```python
from build123d import *

# Parameters (mm, degrees)
BOSS_EXTRUDE1_DEPTH = 45
SKETCH2_R           = 2.75
CUT_EXTRUDE1_DEPTH  = 45
SKETCH3_R           = 5.5
CUT_EXTRUDE2_DEPTH  = 45
CUT_EXTRUDE3_DEPTH  = 45
SKETCH5_R           = 1.6
CUT_EXTRUDE5_DEPTH  = 15
SKETCH6_R           = 1.6
CUT_EXTRUDE6_DEPTH  = 15
FILLET1_R           = 2
FILLET2_R           = 1
FILLET3_R           = 2
FILLET4_R           = 1
SKETCH7_W           = 1
SKETCH7_H           = 92.409175645
CUT_EXTRUDE7_DEPTH  = 45
FILLET8_R           = 2


with BuildPart() as part:
    # Sketch1 → Boss-Extrude1 (new body)
    with BuildSketch(Plane(origin=(0, 0, 0), x_dir=(1, 0, 0), z_dir=(0, 1, 0))):
        with BuildLine():
            Line((-1, 9.949874371), (-1, 44.988887517))
            ThreePointArc((-1, 44.988887517), (-45, 0), (-1, -44.988887517))
            Line((-1, -44.988887517), (-1, -9.949874371))
            ThreePointArc((-1, -9.949874371), (-10, 0), (-1, 9.949874371))
        make_face()
    extrude(amount=BOSS_EXTRUDE1_DEPTH)

    # Sketch2 → Cut-Extrude1 (cut)
    with BuildSketch(Plane(origin=(0, 45, 0), x_dir=(1, 0, 0), z_dir=(0, 1, 0))):
        with Locations(Location((-40, 0, 0), (0, 0, 270))):
            Circle(SKETCH2_R)
        with Locations(Location((-5, 15, 0), (0, 0, 270))):
            Circle(SKETCH2_R)
        with Locations(Location((-5, 40, 0), (0, 0, 270))):
            Circle(SKETCH2_R)
        with Locations(Location((-5, -40, 0), (0, 0, 270))):
            Circle(SKETCH2_R)
    extrude(amount=-CUT_EXTRUDE1_DEPTH, mode=Mode.SUBTRACT)

    # Sketch3 → Cut-Extrude2 (cut)
    with BuildSketch(Plane(origin=(0, 45, 0), x_dir=(1, 0, 0), z_dir=(0, 1, 0))):
        with Locations(Location((-33.5, 6, 0), (0, 0, 270))):
            Circle(SKETCH3_R)
        with Locations(Location((-21.5, 6, 0), (0, 0, 270))):
            Circle(SKETCH3_R)
        with Locations(Location((-11, 21.5, 0), (0, 0, 270))):
            Circle(SKETCH3_R)
        with Locations(Location((-11, 33.5, 0), (0, 0, 270))):
            Circle(SKETCH3_R)
        with Locations(Location((-33.5, -6, 0), (0, 0, 270))):
            Circle(SKETCH3_R)
        with Locations(Location((-21.5, -6, 0), (0, 0, 270))):
            Circle(SKETCH3_R)
        with Locations(Location((-11, -33.5, 0), (0, 0, 270))):
            Circle(SKETCH3_R)
        with Locations(Location((-11, -21.5, 0), (0, 0, 270))):
            Circle(SKETCH3_R)
    extrude(amount=-CUT_EXTRUDE2_DEPTH, mode=Mode.SUBTRACT)

    # Sketch4 → Cut-Extrude3 (cut)
    with BuildSketch(Plane(origin=(0, 45, 0), x_dir=(1, 0, 0), z_dir=(0, 1, 0))):
        with BuildLine():
            ThreePointArc((-11, 43.634848459), (-33.902512538, 29.590870951), (-44.72135955, 5))
            Line((-44.72135955, 5), (-38.908326913, 5))
            ThreePointArc((-38.908326913, 5), (-34.002096593, 11.477033779), (-28, 6))
            ThreePointArc((-28, 6), (-28.022966221, 5.497903407), (-28.091673087, 5))
            Line((-28.091673087, 5), (-27.5, 5))
            Line((-27.5, 5), (-26.908326913, 5))
            ThreePointArc((-26.908326913, 5), (-24.51323898, 10.601129302), (-18.421669276, 10.557837201))
            Line((-18.421669276, 10.557837201), (-14.087297918, 16.948232039))
            ThreePointArc((-14.087297918, 16.948232039), (-16.257600393, 23.11481829), (-11, 27))
            Line((-11, 27), (-11, 28))
            ThreePointArc((-11, 28), (-16.5, 33.5), (-11, 39))
            Line((-11, 39), (-11, 43.634848459))
        make_face()
        with BuildLine():
            Line((-38.908326913, -5), (-44.72135955, -5))
            ThreePointArc((-44.72135955, -5), (-33.902512538, -29.590870951), (-11, -43.634848459))
            Line((-11, -43.634848459), (-11, -39))
            ThreePointArc((-11, -39), (-16.5, -33.5), (-11, -28))
            Line((-11, -28), (-11, -27))
            ThreePointArc((-11, -27), (-16.257600393, -23.11481829), (-14.087297918, -16.948232039))
            Line((-14.087297918, -16.948232039), (-18.421669276, -10.557837201))
            ThreePointArc((-18.421669276, -10.557837201), (-24.51323898, -10.601129302), (-26.908326913, -5))
            Line((-26.908326913, -5), (-27.5, -5))
            Line((-27.5, -5), (-28.091673087, -5))
            ThreePointArc((-28.091673087, -5), (-28.022966221, -5.497903407), (-28, -6))
            ThreePointArc((-28, -6), (-34.002096593, -11.477033779), (-38.908326913, -5))
        make_face()
    extrude(amount=-CUT_EXTRUDE3_DEPTH, mode=Mode.SUBTRACT)

    # Sketch5 → Cut-Extrude5 (cut)
    with BuildSketch(Plane(origin=(-17.521876952, 0, -11.884449008), x_dir=(-0.5613268941159263, 0, 0.8275941746666465), z_dir=(-0.8275941746666464, 0, -0.5613268941159262))):
        with Locations((-2.257852543, 30)):
            Circle(SKETCH5_R)
        with Locations((-2.257852543, 15)):
            Circle(SKETCH5_R)
    extrude(amount=-CUT_EXTRUDE5_DEPTH, mode=Mode.SUBTRACT)

    # Sketch6 → Cut-Extrude6 (cut)
    with BuildSketch(Plane(origin=(-17.521876952, 0, 11.884449008), x_dir=(0.5613268941159263, 0, 0.8275941746666465), z_dir=(-0.8275941746666464, 0, 0.5613268941159262))):
        with Locations((2.257852543, 30)):
            Circle(SKETCH6_R)
        with Locations((2.257852543, 15)):
            Circle(SKETCH6_R)
    extrude(amount=-CUT_EXTRUDE6_DEPTH, mode=Mode.SUBTRACT)

    # Fillet1
    fillet1_edges = [part.edges().sort_by_distance(p)[0] for p in [
        (-18.421669276, 22.5, 10.557837201),
        (-14.087297918, 22.5, 16.948232039),
        (-14.087297918, 22.5, -16.948232039),
        (-18.421669276, 22.5, -10.557837201),
    ]]
    fillet(fillet1_edges, radius=FILLET1_R)

    # Fillet2
    # the kernel refuses this fillet: 1 mm, written as the material it takes off along each edge
    with BuildSketch(Plane(origin=(-11, 47.306540723, 28), x_dir=(0.9970192610334746, 0, 0.0771530500256742), z_dir=(0, -1, 0)), Plane(origin=(-11, 47.306540723, -27), x_dir=(0.9970192610334746, 0, 0.0771530500256742), z_dir=(0, -1, 0))) as fillet2_piece_1:
        with BuildLine():
            CenterArc((0.9258366, -0.997019261), FILLET2_R, 94.424941549, 81.150116902)
            Line((-0.071182661, -0.919866211), (0, 0))
            ThreePointArc((0, 0), (0.424341775, -0.016394064), (0.84868355, 0))
        make_face()
    extrude(amount=49.613081447, mode=Mode.SUBTRACT)
    with BuildSketch(Plane(origin=(-11, 47.306540723, 27), x_dir=(0, 0, 1), z_dir=(0, -1, 0)), Plane(origin=(-11, 47.306540723, -28), x_dir=(0, 0, 1), z_dir=(0, -1, 0))) as fillet2_piece_2:
        with BuildLine():
            CenterArc((0.922616289, -1), FILLET2_R, 90, 81.150116902)
            ThreePointArc((-0.065478524, -0.846153846), (-0.016394064, -0.424341775), (0, 0))
            Line((0, 0), (0.922616289, 0))
        make_face()
    extrude(amount=49.613081447, mode=Mode.SUBTRACT)

    # Fillet3
    fillet3_edges = [part.edges().sort_by_distance(p)[0] for p in [
        (-11, 22.5, 39),
        (-11, 22.5, 43.634848459),
        (-44.72135955, 22.5, 5),
        (-38.908326913, 22.5, 5),
        (-38.908326913, 22.5, -5),
        (-44.72135955, 22.5, -5),
        (-11, 22.5, -43.634848459),
        (-11, 22.5, -39),
    ]]
    fillet(fillet3_edges, radius=FILLET3_R)

    # Fillet4
    # the kernel refuses this fillet: 1 mm, written as the material it takes off along each edge
    with BuildSketch(Plane(origin=(-26.908326913, 46.940828813, 5), x_dir=(-1, 0, 0), z_dir=(0, -1, 0)), Plane(origin=(-28.091673087, 46.940828813, -5), x_dir=(1, 0, 0), z_dir=(0, -1, 0))) as fillet4_piece_1:
        with BuildLine():
            CenterArc((0.776331525, 1), FILLET4_R, 197.920213139, 72.079786861)
            ThreePointArc((-0.175154388, 0.692307692), (-0.076329158, 0.348999608), (0, 0))
            Line((0, 0), (0.776331525, 0))
        make_face()
    extrude(amount=48.881657626, mode=Mode.SUBTRACT)
    with BuildSketch(Plane(origin=(-28.091673087, 46.940828813, 5), x_dir=(-0.24527265600487286, 0, -0.9694541372423533), z_dir=(0, -1, 0)), Plane(origin=(-26.908326913, 46.940828813, -5), x_dir=(0.2452726560048734, 0, 0.9694541372423531), z_dir=(0, -1, 0))) as fillet4_piece_2:
        with BuildLine():
            CenterArc((0.779041242, 0.997890465), FILLET4_R, 194.197947418, 72.079786861)
            Line((-0.190412895, 0.752617809), (0, 0))
            ThreePointArc((0, 0), (0.357060569, 0.011602442), (0.714121139, 0))
        make_face()
    extrude(amount=48.881657626, mode=Mode.SUBTRACT)

    # Sketch7 → Cut-Extrude7 (cut)
    with BuildSketch(Plane(origin=(0, 45, 0), x_dir=(1, 0, 0), z_dir=(0, 1, 0))):
        with Locations((-1.5, -1.215700306)):
            Rectangle(SKETCH7_W, SKETCH7_H)
    extrude(amount=-CUT_EXTRUDE7_DEPTH, mode=Mode.SUBTRACT)

    # Fillet8
    fillet8_edges = [part.edges().sort_by_distance(p)[0] for p in [
        (-2, 22.5, -44.955533586),
        (-2, 22.5, 44.955533586),
        (-2, 22.5, -9.797958971),
        (-2, 22.5, 9.797958971),
    ]]
    fillet(fillet8_edges, radius=FILLET8_R)


solid = part.part
```
Here's how the part is built. I have some questions about the finished solid (model axes, mm). A direction names the side the tool comes from. Give positions to 0.01 mm unless a question says otherwise; leave off trailing zeros. Order: outer loops, then holes, each group sorted by start corner. A loop starts at its lowest first (then second) coordinate and runs counter-clockwise, first axis right, second up. Notation, with made-up numbers: (-33.75, -3.75) - (9.25, -3.75) arc R15 cw to (9.25, 9.25) - close; hole circle Ø8 at (83, 26.5). An arc over 180 degrees is marked (long way). Answer as a JSON object with one key per item and string values. Group by question number.
Item 1: If we section it at C-C on z = -21.5: Please give me the cut outline in (x, y).
Item 2: If we section it at D-D on x = -23: Please give me the cut outline in (y, z).
Item 3: If we mould it in two halves opening along Z, with no side actions, what happens to faces 1 (the flat face through (-16.237, 22.815, 13.779)), 2 (the cylindrical face through (-37.273, 22.815, -0.358)), 3 (the cylindrical face through (-39.29, 22.18, -4.68)), 4 (the cylindrical face through (-17.792, 22.185, -10.776))? For each: pulls with the +Z half, pulls with the -Z half, needs draft (parallel to the pull), parting line crosses it, or undercut.
Item 4: Please list where these lines run through material, in increasing order: probe 1 along Z at (x, y) = (-13.5, 15.5); probe 2 along Z at (x, y) = (-17.5, 39); probe 3 along X at (y, z) = (9, 39).
Item 5: For P1, Ø2, axis at x = -41.5, y = 18.5, coming from the -Z side; P2, Ø6.5, axis at x = -21.5, z = -6, coming from the +Y side; P3, Ø6, axis at y = 38.5, z = 25, coming from the -X side; P4, Ø1.5, axis at x = -28, y = 5.5, coming from the +Z side, each with a flat end and sliding along its axis, tell me the tip position at first contact or that it passes through.
Item 6: Which directions (+Z, -Z, +X, -X, +Y, -Y) give clear straight access to the entire face, cutting with the end or side of a thin tool? Please do faces 5 (the cylindrical face through (-10.58, 22.18, -39.5)), 6 (the cylindrical face through (-6.777, 22.185, -44.487)), 7 (the flat face through (-42, 23, 5)).
Item 7: If we section it at B-B on y = 19: Give the number of separate pieces and of enclosed holes in the cut face, and give its area (3 significant figures).
Item 8: If we section it at A-A on z = 1.5: Please give me the cut outline in (x, y) (3 decimals), and give its area (3 significant figures).
Result set:
{
 "1": {"outline": "(-5.5, 0) - (-2, 0) - (-2, 45) - (-5.5, 45) - close"},
 "2": {"outline": "(0, -0.71) - (45, -0.71) - (45, 0.71) - (0, 0.71) - close"},
 "3": {"face 1": "pulls with the +Z half", "face 2": "undercut", "face 3": "pulls with the -Z half", "face 4": "undercut"},
 "4": {"probe 1": "-16.39 to -13.72, -10.05 to 10.05, 13.72 to 16.39", "probe 2": "-11.91 to -9.82, -2.23 to 2.23, 9.82 to 11.91", "probe 3": "-10.01 to -7.56, -2.44 to -2"},
 "5": {"P1": "z = -5", "P2": "through", "P3": "x = -10.91", "P4": "z = 4.98"},
 "6": {"face 5": "-X, +Y, -Y", "face 6": "-Z, -X, +Y, -Y", "face 7": "+Z, -X, +Y, -Y"},
 "7": {"separate pieces": "1", "enclosed holes": "4", "area": "705 mm²"},
 "8": {"outline": "(-44.975, 0) - (-42.305, 0) - (-42.305, 45) - (-44.975, 45) - close; (-37.695, 0) - (-36.662, 0) - (-36.662, 45) - (-37.695, 45) - close; (-30.338, 0) - (-24.662, 0) - (-24.662, 45) - (-30.338, 45) - close; (-18.338, 0) - (-9.887, 0) - (-9.887, 45) - (-18.338, 45) - close", "area": "802 mm²"}
}
